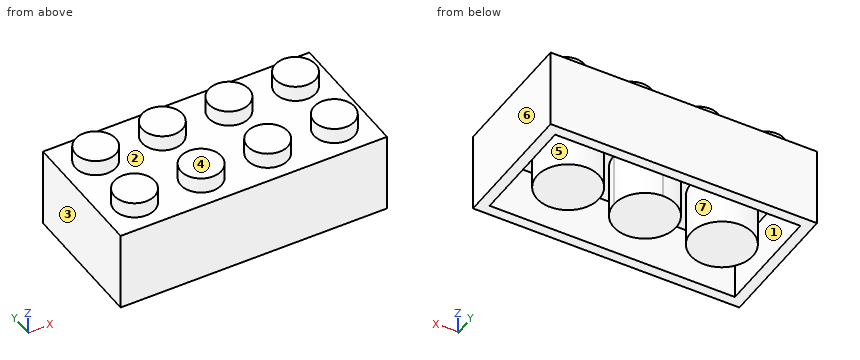
from build123d import *

# Parameters (mm, degrees)
F0_W     = 31.7754
F0_H     = 15.8242
F1_DEPTH = 9.5504
F2_R     = 2.420309
F3_DEPTH = 1.8796
F5_DEPTH = 6.477
F6_R     = 3.709792
F7_DEPTH = 6.477
F8_R     = 1.277131
F9_DEPTH = 0.0508


with BuildPart() as f1:
    # F0 (on Top) → F1 (new body)
    with BuildSketch(Plane.XY):
        Rectangle(F0_W, F0_H)
    extrude(amount=F1_DEPTH)

    # F2 (on face) → F3 (join)
    with BuildSketch(Plane.XY.offset(9.5504)):
        with Locations((-11.915775, 3.95605)):
            Circle(F2_R)
        with Locations((-3.971925, 3.95605)):
            Circle(F2_R)
        with Locations((3.971925, 3.95605)):
            Circle(F2_R)
        with Locations((11.915775, 3.95605)):
            Circle(F2_R)
        with Locations((11.915775, -3.95605)):
            Circle(F2_R)
        with Locations((3.971925, -3.95605)):
            Circle(F2_R)
        with Locations((-3.971925, -3.95605)):
            Circle(F2_R)
        with Locations((-11.915775, -3.95605)):
            Circle(F2_R)
    extrude(amount=F3_DEPTH)

    # F4 (on face) → F5 (cut)
    with BuildSketch(Plane(origin=(0, 0, 0), x_dir=(1, 0, 0), z_dir=(0, 0, -1))):
        Polygon((14.626832, 6.675115), (-12.304062, 6.675115), (-14.626832, 6.675115), (-14.626832, -6.675115), (14.626832, -6.675115), align=None)
    extrude(amount=-F5_DEPTH, mode=Mode.SUBTRACT)

    # F6 (on face) → F7 (join)
    with BuildSketch(Plane(origin=(0, 0, 6.477), x_dir=(1, 0, 0), z_dir=(0, 0, -1))):
        with Locations((-9.168312, 0)):
            Circle(F6_R)
        with BuildLine():
            ThreePointArc((0, -3.709792), (2.623219, -2.623219), (3.709792, 0))
            ThreePointArc((3.709792, 0), (2.623219, 2.623219), (0, 3.709792))
            ThreePointArc((0, 3.709792), (-3.709792, 0), (0, -3.709792))
        make_face()
        with Locations((9.168312, 0)):
            Circle(F6_R)
    extrude(amount=F7_DEPTH)

    # F8 (on face) → F9 (cut)
    with BuildSketch(Plane(origin=(0, 0, 6.477), x_dir=(1, 0, 0), z_dir=(0, 0, -1))):
        with Locations((-12.861121, 4.922554)):
            Circle(F8_R)
        with Locations((-5.436716, 4.922554)):
            Circle(F8_R)
        with Locations((5.436716, 4.922554)):
            Circle(F8_R)
        with Locations((12.861121, 4.922554)):
            Circle(F8_R)
        with Locations((12.861121, -4.922554)):
            Circle(F8_R)
        with Locations((5.436716, -4.922554)):
            Circle(F8_R)
        with Locations((-5.436716, -4.922554)):
            Circle(F8_R)
        with Locations((-12.861121, -4.922554)):
            Circle(F8_R)
    extrude(amount=-F9_DEPTH, mode=Mode.SUBTRACT)


solid = f1.part
Verification items for the finished model (mm, model axes). Face numbers are marked on the shaded views. A direction names the side the tool comes from. Coordinates: 2 decimals unless noted, no trailing zeros. Order: outer loops, then holes, each group sorted by start corner. A loop starts at its lowest first (then second) coordinate and runs counter-clockwise, first axis right, second up. Notation, with made-up numbers: M -25.75,-34 L 29.25,-34 A16 ccw 29.25,-19 Z; hole C 69.25,48 d2. An arc over 180 degrees is marked long. One line per item, written item: value. Start each with the question number.
Item 1: Scan lines: probe 1 along X at (y, z) = (5.25, 6); probe 2 along Y at (x, z) = (-5, 1); probe 3 along Y at (x, z) = (-10, 6). Record each from-to range of solid material in increasing order.
Item 2: Sectioned sample at D-D (x = 6). Enter the section's corners in (y, z), then the cut area to 3 significant figures.
Item 3: Sectioned sample at B-B (x = 10). Enter the section's corners in (y, z).
Item 4: Sectioned sample at A-A (z = 3.5). Enter the section's corners in (x, y).
Item 5: Sectioned sample at C-C (x = 1). Enter the section's corners in (y, z).
Item 6: Access from +Z, -Z, +X, -X, +Y, -Y to the whole of each face (thin tool, end or side, straight path). Record for the marked faces 1, 2 and 3.
Item 7: Gauge pin test, flat end, axial feed: pin 1 (3 mm diameter, centred on x = 5, y = -4.5, fed in from -Z). Record the tip position at first contact, or that the pin passes through.
Item 8: Mould release check, pull along X, two halves, no side actions. Record for the marked faces 4, 5, 6 and 7: released by +X, released by -X, zero draft, split by the parting line, or undercut.
Conclusion:
1. probe 1: x = -15.89 to -14.63, 14.63 to 15.89
1. probe 2: y = -7.91 to -6.68, 6.68 to 7.91
1. probe 3: y = -7.91 to -6.68, -3.62 to 3.62, 6.68 to 7.91
2. outline: M -7.91,0 L -6.68,0 L -6.68,6.48 L -6.07,6.48 L -6.07,6.53 L -3.78,6.53 L -3.78,6.48 L -1.93,6.48 L -1.93,0 L 1.93,0 L 1.93,6.48 L 3.78,6.48 L 3.78,6.53 L 6.07,6.53 L 6.07,6.48 L 6.68,6.48 L 6.68,0 L 7.91,0 L 7.91,9.55 L 5.28,9.55 L 5.28,11.43 L 2.64,11.43 L 2.64,9.55 L -2.64,9.55 L -2.64,11.43 L -5.28,11.43 L -5.28,9.55 L -7.91,9.55 Z
2. area: 99.4 mm^2
3. outline: M -7.91,0 L -6.68,0 L -6.68,6.48 L -3.62,6.48 L -3.62,0 L 3.62,0 L 3.62,6.48 L 6.68,6.48 L 6.68,0 L 7.91,0 L 7.91,9.55 L 5.44,9.55 L 5.44,11.43 L 2.48,11.43 L 2.48,9.55 L -2.48,9.55 L -2.48,11.43 L -5.44,11.43 L -5.44,9.55 L -7.91,9.55 Z
4. outline: M -15.89,-7.91 L 15.89,-7.91 L 15.89,7.91 L -15.89,7.91 Z; C -9.17,0 d7.42; C 0,0 d7.42; C 9.17,0 d7.42; hole M -14.63,-6.68 L 14.63,-6.68 L 14.63,6.68 L -14.63,6.68 Z
5. outline: M -7.91,0 L -6.68,0 L -6.68,6.48 L -3.57,6.48 L -3.57,0 L 3.57,0 L 3.57,6.48 L 6.68,6.48 L 6.68,0 L 7.91,0 L 7.91,9.55 L -7.91,9.55 Z
6. face 1: -Z
6. face 2: +Z
6. face 3: +Z, -Z, -X, +Y, -Y
7. pin 1: stops at z = 6.48
8. face 4: zero draft
8. face 5: undercut
8. face 6: released by +X
8. face 7: undercut
